Autodesk Inventor part; units mm, degrees
ref_plane "YZ Plane" through (0, 0, 0) normal (1, 0, 0) x (0, 1, 0)
ref_plane "XZ Plane" through (0, 0, 0) normal (0, 1, 0) x (-1, 0, 0)
ref_plane "XY Plane" through (0, 0, 0) normal (0, 0, 1) x (1, 0, 0)
ref_plane "Płaszczyzna konstrukcyjna1" through (0, 0, 0) normal (0, 0, 1) x (1, 0, 0)
sketch "Szkic1" plane through (0, 0, 0) normal (0, 0, 1) x (1, 0, 0)
  circle A0 centre (110, 0) radius 110
  circle A1 centre (110, 0) radius 140
  point P0 (0, 0)
extrude "Wyciągnięcie proste1" add sketch "Szkic1" along normal blind 310 contours A0 | A1
fillet "Zaokrąglenie1" radius 30 1 edges at (-30, 0, 0)
sketch "Szkic2" plane through (110, 0, 310) normal (0, 0, 1) x (1, 0, 0)
  circle A0 centre (0, 0) radius 80
  circle A1 centre (0, 0) radius 140
  point P0 (-110, 0)
  dimension "d3" = 160
extrude "Wyciągnięcie proste2" cut sketch "Szkic2" against normal blind 30
fillet "Zaokrąglenie2" radius 30 1 edges at (-30, 0, 280)
fillet "Zaokrąglenie3" radius 20 1 edges at (30, 0, 280)
sketch "Szkic3" plane through (110, 0, 310) normal (0, 0, 1) x (1, 0, 0)
  circle A0 centre (0, 0) radius 32.5
  point P0 (-110, 0)
  dimension "d8" = 65
extrude "Wyciągnięcie proste3" cut sketch "Szkic3" against normal blind 123
chamfer "Faza1" distance 1 angle 45 1 edges at (77.5, 0, 187)
properties part number "wodaxD" material "Woda"
The listing builds one solid part. Answer for the finished solid, in the listing's coordinates (mm). A direction names the side the tool comes from. Give positions to 0.01 mm unless a question says otherwise; leave off trailing zeros. Loops run counter-clockwise (first coordinate to the right, second up) from the corner with the lowest first, then second, coordinate; pieces in that order, holes last. Notation, with made-up numbers: M -17.5,-35.75 L 6.5,-35.75 A23 cw 6.5,-9.75 Z; hole C 41,-17.75 d11. An arc over 180 degrees is marked long. One line per item, written item: value.
Q1. Flat-ended cylindrical pins translate along their axes: P1, Ø8, axis at x = 180.5, y = -100.5, coming from the +Z side; P2, Ø5, axis at y = -51.5, z = 55.5, coming from the +X side; P3, Ø2, axis at y = -108, z = 206.5, coming from the -X side; P4, Ø1, axis at x = 146, y = -83, coming from the -Z side. Find the tip coordinate at first contact, or state that the pin passes through.
Working result:
P1: stops at z = 278.69
P2: stops at x = 241.14
P3: stops at x = 19.72
P4: stops at z = 0
Q2. A cutting plane is placed at A-A on y = 0. Determine the outline of the cut face in (x, z).
Working result:
outline: M -30,30 A30 ccw 0,0 L 220,0 A30 ccw 250,30 L 250,250 A30 ccw 220,280 L 210,280 A20 cw 190,300 L 190,310 L 142.5,310 L 142.5,188 L 141.5,187 L 78.5,187 L 77.5,188 L 77.5,310 L 30,310 L 30,300 A20 cw 10,280 L 0,280 A30 ccw -30,250 Z
Q3. For faces 1 (the face through (141, 9.76, 249.85)), 2 (the face through (108, 2, 0)), determine the directions among +Z, -Z, +X, -X, +Y, -Y from which every point of the face is accessible in a straight line to the end or side of a thin tool.
Working result:
face 1: +Z
face 2: -Z, +X, -X, +Y, -Y
Q4. Find the intervals of material crossed by line 1 (Y direction, x = 110, z = 215); line 2 (Y direction, x = 110, z = 284); line 3 (Z direction, x = 25, y = 58.5), in increasing order. Write a range as from..to.
Working result:
line 1: y = -140..-32.5, 32.5..140
line 2: y = -88..-32.5, 32.5..88
line 3: z = 0..280
Q5. A cutting plane is placed at C-C on z = 48.5. Determine the outline of the cut face in (x, y).
Working result:
outline: C 110,0 d280
Q6. A cutting plane is placed at B-B on x = 110. Determine the outline of the cut face in (y, z).
Working result:
outline: M -140,30 A30 ccw -110,0 L 110,0 A30 ccw 140,30 L 140,250 A30 ccw 110,280 L 100,280 A20 cw 80,300 L 80,310 L 32.5,310 L 32.5,188 L 31.5,187 L -31.5,187 L -32.5,188 L -32.5,310 L -80,310 L -80,300 A20 cw -100,280 L -110,280 A30 ccw -140,250 Z
Q7. Determine the mould class of faces 3 (the face through (110, 0, 187)), 4 (the face through (144, 1, 310)), 5 (the face through (174.601, 124.204, 138.46)) for opening direction Y: +Y half, -Y half, draft (parallel to the pull), parting line (faces both ways), or undercut.
Working result:
face 3: undercut
face 4: draft
face 5: parting line
